Read the model definition and answer for the solid it produces. Units are mm, in the model's axes. A direction names the side the tool comes from. Give positions to 0.01 mm unless a question says otherwise; leave off trailing zeros. Loops run counter-clockwise (first coordinate to the right, second up) from the corner with the lowest first, then second, coordinate; pieces in that order, holes last. Notation, with made-up numbers: (-25, 3.5) -> (7, 3.5) arc R19 ccw to (7, 29.5) -> close; hole circle Ø11 at (80.25, -36). An arc over 180 degrees is marked (long way). Answer as CSV lines item,"result". Start each with the question number.
```python
from build123d import *

# Parameters (mm, degrees)
F0_W     = 250
F0_H     = 158
F0_R     = 1.2
F0_W_2   = 120
F0_H_2   = 100
F1_DEPTH = 3
F2_R     = 5


with BuildPart() as f1:
    # F0 (on Top) → F1 (new body)
    with BuildSketch(Plane.XY):
        Rectangle(F0_W, F0_H)
        with BuildLine():
            ThreePointArc((-89.5, -66), (-86.5, -69), (-89.5, -72))
            Line((-89.5, -72), (-110.5, -72))
            ThreePointArc((-110.5, -72), (-113.5, -69), (-110.5, -66))
            Line((-110.5, -66), (-89.5, -66))
        make_face(mode=Mode.SUBTRACT)
        with Locations((-75, -66.5)):
            Circle(F0_R, mode=Mode.SUBTRACT)
        with Locations((-112.5, -55)):
            Circle(F0_R, mode=Mode.SUBTRACT)
        with Locations((-45, -66.5)):
            Circle(F0_R, mode=Mode.SUBTRACT)
        with Locations((-112.5, -25)):
            Circle(F0_R, mode=Mode.SUBTRACT)
        with Locations((45, -66.5)):
            Circle(F0_R, mode=Mode.SUBTRACT)
        with Locations((75, -66.5)):
            Circle(F0_R, mode=Mode.SUBTRACT)
        with BuildLine():
            ThreePointArc((89.5, -72), (86.5, -69), (89.5, -66))
            Line((89.5, -66), (110.5, -66))
            ThreePointArc((110.5, -66), (113.5, -69), (110.5, -72))
            Line((110.5, -72), (89.5, -72))
        make_face(mode=Mode.SUBTRACT)
        with Locations((112.5, -55)):
            Circle(F0_R, mode=Mode.SUBTRACT)
        with Locations((112.5, -25)):
            Circle(F0_R, mode=Mode.SUBTRACT)
        with Locations((-112.5, 25)):
            Circle(F0_R, mode=Mode.SUBTRACT)
        with Locations((-112.5, 55)):
            Circle(F0_R, mode=Mode.SUBTRACT)
        with BuildLine():
            ThreePointArc((-89.5, 72), (-86.5, 69), (-89.5, 66))
            Line((-89.5, 66), (-110.5, 66))
            ThreePointArc((-110.5, 66), (-113.5, 69), (-110.5, 72))
            Line((-110.5, 72), (-89.5, 72))
        make_face(mode=Mode.SUBTRACT)
        with Locations((-75, 66.5)):
            Circle(F0_R, mode=Mode.SUBTRACT)
        with Locations((-45, 66.5)):
            Circle(F0_R, mode=Mode.SUBTRACT)
        Rectangle(F0_W_2, F0_H_2, mode=Mode.SUBTRACT)
        with Locations((112.5, 25)):
            Circle(F0_R, mode=Mode.SUBTRACT)
        with Locations((45, 66.5)):
            Circle(F0_R, mode=Mode.SUBTRACT)
        with Locations((112.5, 55)):
            Circle(F0_R, mode=Mode.SUBTRACT)
        with Locations((75, 66.5)):
            Circle(F0_R, mode=Mode.SUBTRACT)
        with BuildLine():
            ThreePointArc((110.5, 72), (113.5, 69), (110.5, 66))
            Line((110.5, 66), (89.5, 66))
            ThreePointArc((89.5, 66), (86.5, 69), (89.5, 72))
            Line((89.5, 72), (110.5, 72))
        make_face(mode=Mode.SUBTRACT)
    extrude(amount=F1_DEPTH)

    # F2
    f2_edges = [f1.edges().sort_by_distance(p)[0] for p in [
        (-60, 50, 1.5),
        (-60, -50, 1.5),
        (60, -50, 1.5),
        (60, 50, 1.5),
    ]]
    fillet(f2_edges, radius=F2_R)


solid = f1.part
```
(1) Find the intervals of material crossed by line 1 along Y through (x, z) = (-75, 2.25); line 2 along Y through (x, z) = (111, 0.4); line 3 along Y through (x, z) = (-45, 0.8), in increasing order. Write a range as from..to.
(2) A tool of negligible diameter and unlimited length cuts with its end or side. For faces 1 (the face through (58, -49, 2)), 2 (the face through (-2, 54, 3)), from which of +Z, -Z, +X, -X, +Y, -Y can it reach the whole face along a straight path? Write none if from no direction.
(3) Find section B-B on x = -30.5. Write down the section's boundary in (y, z).
(4) Find section C-C on z = 2.2. Give the number of separate pieces and of enclosed holes in the cut face, then the cut area to 3 significant figures.
(5) The mould has two halves that part along Y. Classify faces 3 (the face through (-2, 54, 0)), 4 (the face through (-59, 48, 2)): pulls with the +Y half, pulls with the -Y half, needs draft (parallel to the pull), parting line crosses it, or undercut.
(6) Find section A-A on y = -37.5. Write down the section's boundary in (x, z), then the cut area to 3 significant figures.
Answer block:
1,line 1,"y = -79..-67.7, -65.3..65.3, 67.7..79"
1,line 2,"y = -79..-71.96, -66.04..66.04, 71.96..79"
1,line 3,"y = -79..-67.7, -65.3..-50, 50..65.3, 67.7..79"
2,face 1,"+Z, -Z"
2,face 2,"+Z, +X, -X, +Y, -Y"
3,outline,"(-79, 0) -> (-50, 0) -> (-50, 3) -> (-79, 3) -> close; (50, 0) -> (79, 0) -> (79, 3) -> (50, 3) -> close"
4,separate pieces,"1"
4,enclosed holes,"21"
4,area,"26,800 mm2"
5,face 3,"needs draft"
5,face 4,"undercut"
6,outline,"(-125, 0) -> (-60, 0) -> (-60, 3) -> (-125, 3) -> close; (60, 0) -> (125, 0) -> (125, 3) -> (60, 3) -> close"
6,area,"390 mm2"
